The listing builds one solid part. Answer for the finished solid, in the listing's coordinates (mm). A direction names the side the tool comes from. Round coordinates to 2 decimals unless told otherwise and drop trailing zeros. Write each loop counter-clockwise with the first axis right and the second up, starting at its lowest first coordinate (ties: lowest second). Pieces come first, ordered by that corner, then holes.
Item 1: For a pull along X with two mould halves and no side action, classify faces 1 (the face through (23, -3, 6)), 2 (the face through (10, 2, -6.65)), 3 (the face through (0.2, 6.35, -0.17)) as +X half, -X half, draft (parallel to the pull), parting line (faces both ways), or undercut.
Item 2: Find section B-B on x = 29. Give the vertices of the cut face in (y, z), then the cut area to 3 significant figures.
Item 3: Each of these flat-tipped pins is pushed along its axis until it touches: pin 1 (6.5 mm diameter, centred on x = 2, y = 3, fed in from +Z); pin 2 (4.5 mm diameter, centred on x = 18.5, z = -7, fed in from +Y); pin 3 (7.5 mm diameter, centred on x = 27.5, z = 5.5, fed in from +Y); pin 4 (6.5 mm diameter, centred on y = -2.5, z = -5, fed in from -X). Where does it stop, or does it pass through?
Item 4: Find the intervals of material crossed by probe 1 along Z at (x, y) = (14.5, 7.25); probe 2 along Y at (x, z) = (4.2, 0); probe 3 along Y at (x, z) = (15, -4.5), in increasing order.
Item 5: Find section A-A on x = 24.5. Give the vertices of the cut face in (y, z), then the cut area to 3 significant figures.
Item 6: A tool of negligible diameter and unlimited length cuts with its end or side. For faces 4 (the face through (14.724, 10.197, -8.374)), 5 (the face through (17, -2, 0)), 6 (the face through (19, 1.3, -10.3)), 7 (the face through (22, -5, -1.588)), 8 (the face through (10, 2, -10.05)), from which of +Z, -Z, +X, -X, +Y, -Y can it reach the whole face along a straight path? Write none if from no direction.
```python
from build123d import *

# Parameters (mm, degrees)
SKETCH2_W           = 21.7
SKETCH2_H           = 25.05
SKETCH2_RX          = 9.525
SKETCH2_RY          = 6.35
BOSS_EXTRUDE1_DEPTH = 12.7
SKETCH3_W           = 21.660653916
SKETCH3_H           = 25.05
BOSS_EXTRUDE2_DEPTH = 3
SKETCH5_W           = 18.892037138
SKETCH5_H           = 21.7
BOSS_EXTRUDE3_DEPTH = 2
SKETCH6_W           = 30
SKETCH6_H           = 21.7
BOSS_EXTRUDE4_DEPTH = 4
SKETCH7_W           = 21.7
SKETCH7_H           = 1
SKETCH7_W_2         = 3.175
SKETCH7_H_2         = 3
CUT_EXTRUDE2_DEPTH  = 23
SKETCH7_3_W         = 21.7
SKETCH7_3_H         = 7.272473706
CUT_EXTRUDE3_DEPTH  = 44.803879418
SKETCH11_R          = 1
CUT_EXTRUDE8_DEPTH  = 33.487034031
CUT_EXTRUDE4_REACH  = 47.088
SKETCH9_R           = 1
SKETCH15_W          = 3.4
SKETCH15_H          = 3.4
CUT_EXTRUDE9_DEPTH  = 28.443249332
FILLET5_R           = 6.35
FILLET6_R           = 2
FILLET7_R           = 2


with BuildPart() as part:
    # Sketch2 → Boss-Extrude1 (new body)
    with BuildSketch(Plane(origin=(16.497783942, 9.525, 0), x_dir=(0, 0, -1), z_dir=(0.8660254037844379, 0.5000000000000013, 0))):
        Rectangle(SKETCH2_W, SKETCH2_H)
        with Locations(Location((0, 0), (0, 0, 90))):
            Ellipse(SKETCH2_RX, SKETCH2_RY, mode=Mode.SUBTRACT)
    extrude(amount=-BOSS_EXTRUDE1_DEPTH)

    # Sketch3 → Boss-Extrude2 (add)
    with BuildSketch(Plane(origin=(5.499261314, 3.175, 0), x_dir=(0, 0, 1), z_dir=(-0.8660254037844379, -0.5000000000000014, 0))):
        with Locations((-0.019673042, 0)):
            Rectangle(SKETCH3_W, SKETCH3_H)
    extrude(amount=BOSS_EXTRUDE2_DEPTH)

    # Sketch5 → Boss-Extrude3 (add)
    with BuildSketch(Plane(origin=(0, 0, 0), x_dir=(-1, 0, 0), z_dir=(0, 1, 0))):
        with Locations((-13.314265373, 0)):
            Rectangle(SKETCH5_W, SKETCH5_H)
    extrude(amount=-BOSS_EXTRUDE3_DEPTH)

    # Sketch6 → Boss-Extrude4 (add)
    with BuildSketch(Plane.XZ.offset(2)):
        with Locations((18.868246804, 0)):
            Rectangle(SKETCH6_W, SKETCH6_H)
    extrude(amount=BOSS_EXTRUDE4_DEPTH)

    # Sketch7 → Cut-Extrude2 (cut)
    with BuildSketch(Plane(origin=(33.868246804, 0, 0), x_dir=(0, 0, -1), z_dir=(1, 0, 0))):
        with Locations((0, -2.5)):
            Rectangle(SKETCH7_W, SKETCH7_H)
        with Locations((0, -4.5)):
            Rectangle(SKETCH7_W_2, SKETCH7_H_2)
    extrude(amount=-CUT_EXTRUDE2_DEPTH, mode=Mode.SUBTRACT)

    # Sketch7<3> → Cut-Extrude3 (cut, through all)
    with BuildSketch(Plane(origin=(33.868246804, 0, 0), x_dir=(0, 0, -1), z_dir=(1, 0, 0))):
        with Locations((0, -9.636236853)):
            Rectangle(SKETCH7_3_W, SKETCH7_3_H)
    extrude(amount=-CUT_EXTRUDE3_DEPTH, mode=Mode.SUBTRACT)

    # Sketch11 → Cut-Extrude8 (cut, through all)
    with BuildSketch(Plane(origin=(19.672783942, 0.194872981, 0), x_dir=(0, 0, -1), z_dir=(-1, 0, 0))):
        with Locations(Location((0, -3.830865705, 0), (0, 0, 90))):
            Circle(SKETCH11_R)
    extrude(amount=CUT_EXTRUDE8_DEPTH, mode=Mode.SUBTRACT)

    # Sketch9 → Cut-Extrude4 (cut, up to next)
    with BuildSketch(Plane(origin=(0, 0, -10.85), x_dir=(-1, 0, 0), z_dir=(0, 0, -1)), mode=Mode.PRIVATE) as cut_extrude4_sk1:
        with Locations((-14.332720433, 8.275)):
            Circle(SKETCH9_R)
    cut_extrude4_tool1 = extrude(cut_extrude4_sk1.sketch, amount=-CUT_EXTRUDE4_REACH, mode=Mode.PRIVATE) & part.part
    cut_extrude4 = cut_extrude4_tool1.solids().sort_by_distance((14.33272, 8.275, -10.85))[0]
    add(cut_extrude4, mode=Mode.SUBTRACT)

    # Sketch15 → Cut-Extrude9 (cut, symmetric)
    with BuildSketch(Plane(origin=(16.497783942, 9.525, 0), x_dir=(0.7757354378747654, -0.6310582623064579, 0), z_dir=(0.6310582623064579, 0.7757354378747654, 0))):
        with Locations((-0.1, -8.35)):
            Rectangle(SKETCH15_W, SKETCH15_H)
    cut_extrude9 = extrude(amount=CUT_EXTRUDE9_DEPTH, both=True, mode=Mode.SUBTRACT)

    # Mirror1: Cut-Extrude4, Cut-Extrude9 across plane
    add(cut_extrude4.mirror(Plane.XY), mode=Mode.SUBTRACT)
    add(cut_extrude9.mirror(Plane.XY), mode=Mode.SUBTRACT)

    # Fillet5
    fillet5_edges = [part.edges().sort_by_distance(p)[0] for p in [
        (33.868246804, -4.5, 10.85),
        (33.868246804, -4.5, -10.85),
        (22.760283942, -1, -10.85),
        (22.760283942, -1, 10.85),
        (4.736022628, 17.196968182, 10.85),
        (3.436984522, 16.446968182, -10.85),
    ]]
    fillet(fillet5_edges, radius=FILLET5_R)

    # Fillet6
    fillet6_edges = [part.edges().sort_by_distance(p)[0] for p in [
        (33.868246804, -4.5, 1.5875),
        (33.868246804, -4.5, -1.5875),
    ]]
    fillet(fillet6_edges, radius=FILLET6_R)

    # Fillet7
    # the kernel refuses this fillet: 2 mm, written as the material it takes off along each edge
    with BuildSketch(Plane(origin=(22.760283942, 0, 8.429393602), x_dir=(-1, 0, 0), z_dir=(0, 0, -1))) as fillet7_piece_1:
        with BuildLine():
            CenterArc((2, -1.571757441), FILLET7_R, 128.197977663, 51.802022337)
            Line((0, -1.571757441), (-0.04, -1.571757441))
            Line((-0.04, -1.571757441), (-0.04, 0))
            Line((-0.04, 0), (0, 0.04))
            ThreePointArc((0, 0.04), (0.381619343, 0.04), (0.73850346, 0.031435149))
            Line((0.73850346, 0.031435149), (0.763238686, 0))
        make_face()
    extrude(amount=16.858787203, mode=Mode.SUBTRACT)


solid = part.part
```
Check values:
1. face 1: draft
1. face 2: undercut
1. face 3: -X half
2. outline: (-6, -10.67) - (-3, -10.67) - (-3, -1.59) - (-6, -1.59) - close; (-6, 1.59) - (-3, 1.59) - (-3, 10.67) - (-6, 10.67) - close
2. area: 54.5 mm2
3. pin 1: stops at z = 10.85
3. pin 2: stops at y = 9.91
3. pin 3: stops at y = -3
3. pin 4: stops at x = 3.44
4. probe 1: z = -10.85 to -10.05, -6.65 to -6.32, 6.32 to 6.65, 10.05 to 10.85
4. probe 2: y = -6 to 3.03, 5.03 to 5.43, 13.42 to 16.89
4. probe 3: y = -6 to -3, -2 to 0.9
5. outline: (-6, -10.85) - (-3, -10.85) - (-3, -1.59) - (-6, -1.59) - close; (-6, 1.59) - (-3, 1.59) - (-3, 10.85) - (-6, 10.85) - close
5. area: 55.6 mm2
6. face 4: +X
6. face 5: +Z, -Z, +X
6. face 6: -Z, +X, +Y
6. face 7: +X, -Y
6. face 8: none
